Here's how the part is built. I have some questions about the finished solid (model axes, mm). Face numbers are marked on the shaded views. Give positions to 0.01 mm unless a question says otherwise; leave off trailing zeros. Write each loop counter-clockwise with the first axis right and the second up, starting at its lowest first coordinate (ties: lowest second). Pieces come first, ordered by that corner, then holes. Notation, with made-up numbers: (64, 20) -> (90, 20) arc R23 cw to (90, 50) -> close; hole circle Ø9 at (-30.5, 45). An arc over 180 degrees is marked (long way). Put each result on its own line as item: value. Start each with the question number.
from build123d import *

# Parameters (mm, degrees)
F0_R     = 76.2
F1_DEPTH = 28.575
F2_R     = 7.9375
F3_DEPTH = 25.4


with BuildPart() as f1:
    # F0 (on Top) → F1 (new body)
    with BuildSketch(Plane.XY):
        Circle(F0_R)
    extrude(amount=F1_DEPTH)

    # F2 (on face) → F3 (cut)
    with BuildSketch(Plane.XY.offset(28.575)):
        with Locations((-30.6127599113, 36.4828666035)):
            Circle(F2_R)
        with Locations((-57.7422437973, 33.3375)):
            Circle(F2_R)
        with Locations((-42.8578638759, 51.076013245)):
            Circle(F2_R)
        with Locations((-22.8041930562, 62.6540054909)):
            Circle(F2_R)
        with Locations((0, 66.675)):
            Circle(F2_R)
        with Locations((0, 47.625)):
            Circle(F2_R)
        with Locations((0, 28.575)):
            Circle(F2_R)
        with Locations((-18.3676559468, 21.8897199621)):
            Circle(F2_R)
        with Locations((-28.1408815423, 4.9619966768)):
            Circle(F2_R)
        with Locations((-46.9014692372, 8.2699944614)):
            Circle(F2_R)
        with Locations((-65.6620569321, 11.5779922459)):
            Circle(F2_R)
        with Locations((-65.6620569321, -11.5779922459)):
            Circle(F2_R)
        with Locations((-57.7422437973, -33.3375)):
            Circle(F2_R)
        with Locations((-41.2444598552, -23.8125)):
            Circle(F2_R)
        with Locations((-24.7466759131, -14.2875)):
            Circle(F2_R)
        with Locations((-8.7988181024, -5.08)):
            Circle(F2_R)
        with Locations((-9.7732255955, -26.851716639)):
            Circle(F2_R)
        with Locations((-16.2887093259, -44.7528610649)):
            Circle(F2_R)
        with Locations((-22.8041930562, -62.6540054909)):
            Circle(F2_R)
        with Locations((-42.8578638759, -51.076013245)):
            Circle(F2_R)
        with Locations((0, -66.675)):
            Circle(F2_R)
        with Locations((22.8041930562, -62.6540054909)):
            Circle(F2_R)
        with Locations((16.2887093259, -44.7528610649)):
            Circle(F2_R)
        with Locations((9.7732255955, -26.851716639)):
            Circle(F2_R)
        with Locations((8.7988181024, -5.08)):
            Circle(F2_R)
        with Locations((0, 10.16)):
            Circle(F2_R)
        with Locations((18.3676559468, 21.8897199621)):
            Circle(F2_R)
        with Locations((30.6127599113, 36.4828666035)):
            Circle(F2_R)
        with Locations((42.8578638759, 51.076013245)):
            Circle(F2_R)
        with Locations((22.8041930562, 62.6540054909)):
            Circle(F2_R)
        with Locations((57.7422437973, 33.3375)):
            Circle(F2_R)
        with Locations((65.6620569321, 11.5779922459)):
            Circle(F2_R)
        with Locations((46.9014692372, 8.2699944614)):
            Circle(F2_R)
        with Locations((28.1408815423, 4.9619966768)):
            Circle(F2_R)
        with Locations((24.7466759131, -14.2875)):
            Circle(F2_R)
        with Locations((41.2444598552, -23.8125)):
            Circle(F2_R)
        with Locations((65.6620569321, -11.5779922459)):
            Circle(F2_R)
        with Locations((57.7422437973, -33.3375)):
            Circle(F2_R)
        with Locations((42.8578638759, -51.076013245)):
            Circle(F2_R)
    extrude(amount=-F3_DEPTH, mode=Mode.SUBTRACT)


solid = f1.part
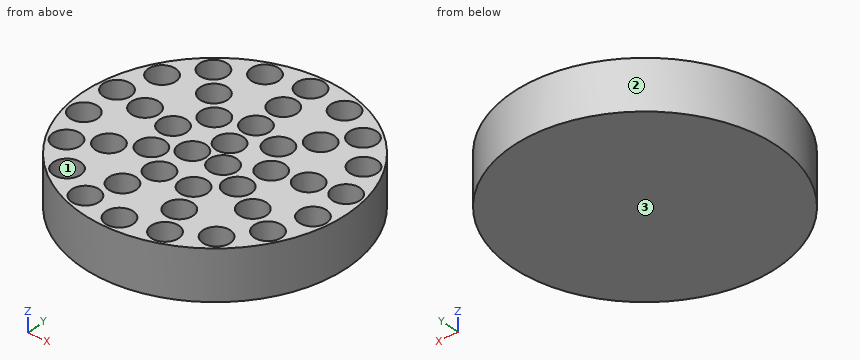
1) I want a section at B-B, the plane z = 8. State how many separate pieces and enclosed holes the cut face has, and give its area (3 significant figures).
2) I want a section at A-A, the plane x = 53. Write out the boundary of the cut face in (y, z) (3 decimals), and give its area (3 significant figures).
3) I'm going to push flat-ended pins straight in: pin 1 Ø4 at (y, z) = (-45, 9) entering from -X; pin 2 Ø8 at (x, y) = (-32, 34.5) entering from +Z (3 decimals); pin 3 Ø12 at (x, z) = (-42, 22) entering from +Y. Where does each tip first touch, or does it pass through?
4) I need wall thicknesses on probe 1 along Y at (x, z) = (44, 14.75); probe 2 along X at (y, z) = (66.5, 18); probe 3 along Y at (x, z) = (32, 25.25). Which ranges of each line are inside material? Lowest first, please.
5) Thinking about a two-plate mould opening in Y: for the marked faces 1, 2 and 3, which applies, released by +Y, released by -Y, zero draft, split by the parting line, or undercut?
Established:
1. separate pieces: 1
1. enclosed holes: 39
1. area: 10,500 mm2
2. outline: (-54.749, 0) -> (54.749, 0) -> (54.749, 28.575) -> (39.703, 28.575) -> (39.703, 3.175) -> (26.972, 3.175) -> (26.972, 28.575) -> (13.351, 28.575) -> (13.351, 3.175) -> (3.189, 3.175) -> (3.189, 28.575) -> (-26.972, 28.575) -> (-26.972, 3.175) -> (-39.703, 3.175) -> (-39.703, 28.575) -> (-54.749, 28.575) -> close
2. area: 2,220 mm2
3. pin 1: stops at x = -62.91
3. pin 2: stops at z = 3.175
3. pin 3: stops at y = 67.16
4. probe 1: y = -62.21 to -58.93, -43.22 to -31.26, -16.37 to 0.88, 15.66 to 43.22, 58.93 to 62.21
4. probe 2: x = -37.2 to -29.75, -15.86 to -7.94, 7.94 to 15.86, 29.75 to 37.2
4. probe 3: y = -69.16 to -17.51, -11.06 to -1.97, 11.9 to 28.67, 44.3 to 69.16
5. face 1: undercut
5. face 2: split by the parting line
5. face 3: zero draft
